Verification items for the finished model (mm, model axes). A direction names the side the tool comes from. Coordinates: 2 decimals unless noted, no trailing zeros. Loops run counter-clockwise (first coordinate to the right, second up) from the corner with the lowest first, then second, coordinate; pieces in that order, holes last. Notation, with made-up numbers: (11.5, -28.5) -> (16.5, -28.5) arc R20 ccw to (16.5, -2.5) -> close; hole circle Ø1 at (61.25, 42). An arc over 180 degrees is marked (long way). Answer as a JSON object with one key per item and string values. Group by question number.
Q1. Release check for a two-part mould opening along Y. For faces 1 (the flat face through (12, -8.029, -35)), 2 (the flat face through (42.52, -20, -20)), 3 (the flat face through (11, 0, -24)) record: released by +Y, released by -Y, zero draft, split by the parting line, or undercut.
Q2. Cross-section at A-A on z = -35. Record the boundary of the cut face in (x, y).
Q3. Cross-section at C-C on y = -4.5. Record the boundary of the cut face in (x, z), and give its area (3 significant figures).
Q4. Set-up check for faces 4 (the flat face through (-10, -16, -14.326)), 5 (the flat face through (12, -17, -30.785)), 6 (the flat face through (-19.554, -16, -24)), 7 (the flat face through (30.772, -7, -7)): record each of +Z, -Z, +X, -X, +Y, -Y from which the full face is reachable in a straight line by a thin tool's end or side.
Q5. Gauge pin test, flat ends, axial feed: pin 1 Ø3.5 at (x, z) = (39, -4) entering from +Y; pin 2 Ø5.5 at (x, y) = (4, -13.5) entering from -Z; pin 3 Ø11.5 at (y, z) = (-22, -3.5) entering from -X. Record the tip position at first contact, or that the pin passes through.
Q6. Cross-section at B-B on x = 27. Record the boundary of the cut face in (y, z), and give its area (3 significant figures).
Q7. Scan lines: L1, parallel to Y at x = 25.5, z = -38; L2, parallel to Z at x = -6.5, y = -23; L3, parallel to Z at x = 10.5, y = -12.5. Record each from-to range of solid material in increasing order.
Q8. Cross-section at D-D on z = -10. Record the boundary of the cut face in (x, y), and give its area (3 significant figures).
```python
from build123d import *

# Parameters (mm, degrees)
F1_DEPTH = 33.274
F2_W     = 11.7478076556
F2_H     = 13.536944912
F3_DEPTH = 14.986
F4_W     = 17.6784005016
F4_H     = 8.8392011821
F5_DEPTH = 84.836


with BuildPart() as f1:
    # F0 (on Front) → F1 (new body)
    with BuildSketch(Plane.XZ):
        Polygon((42.5196029246, 0), (0, 0), (0, -14.3256001174), (-19.5541083813, -14.3256001174), (-19.5541083813, -39.6240018308), (42.5196029246, -39.6240018308), align=None)
    extrude(amount=F1_DEPTH)

    # F2 (on face) → F3 (cut)
    with BuildSketch(Plane.XY):
        with Locations((36.6456990968, -6.768472456)):
            Rectangle(F2_W, F2_H)
    extrude(amount=-F3_DEPTH, mode=Mode.SUBTRACT)

    # F4 (on face) → F5 (cut)
    with BuildSketch(Plane.YZ.offset(42.5196029246)):
        with Locations((-16.8679049239, -35.2044012398)):
            Rectangle(F4_W, F4_H)
    extrude(amount=-F5_DEPTH, mode=Mode.SUBTRACT)


solid = f1.part
```
Computed values:
{
 "1": {"face 1": "undercut", "face 2": "zero draft", "face 3": "released by +Y"},
 "2": {"outline": "(-19.55, -33.27) -> (42.52, -33.27) -> (42.52, -25.71) -> (-19.55, -25.71) -> close; (-19.55, -8.03) -> (42.52, -8.03) -> (42.52, 0) -> (-19.55, 0) -> close"},
 "3": {"outline": "(-19.55, -39.62) -> (42.52, -39.62) -> (42.52, -14.99) -> (30.77, -14.99) -> (30.77, 0) -> (0, 0) -> (0, -14.33) -> (-19.55, -14.33) -> close", "area": "2,000 mm²"},
 "4": {"face 4": "+Z, -X, +Y, -Y", "face 5": "-Z, +X, -X", "face 6": "+Z, -Z, -X, +Y, -Y", "face 7": "+Z, +X, +Y"},
 "5": {"pin 1": "stops at y = -13.54", "pin 2": "stops at z = -30.78", "pin 3": "stops at x = 0"},
 "6": {"outline": "(-33.27, -39.62) -> (-25.71, -39.62) -> (-25.71, -30.78) -> (-8.03, -30.78) -> (-8.03, -39.62) -> (0, -39.62) -> (0, 0) -> (-33.27, 0) -> close", "area": "1,160 mm²"},
 "7": {"L1": "y = -33.27 to -25.71, -8.03 to 0", "L2": "z = -30.78 to -14.33", "L3": "z = -30.78 to 0"},
 "8": {"outline": "(0, -33.27) -> (42.52, -33.27) -> (42.52, -13.54) -> (30.77, -13.54) -> (30.77, 0) -> (0, 0) -> close", "area": "1,260 mm²"}
}
